Verification items for the finished model (mm, model axes). Coordinates: 2 decimals unless noted, no trailing zeros. Loops run counter-clockwise (first coordinate to the right, second up) from the corner with the lowest first, then second, coordinate; pieces in that order, holes last. Notation, with made-up numbers: (-18.75, -23) - (31.25, -23) arc R20 cw to (31.25, 1) - close; hole circle Ø5 at (41, 14.25). An arc over 180 degrees is marked (long way). One line per item, written item: value. Start each with the question number.
(1) Section check A-A (y = 74.5). Record the boundary of the cut face in (x, z).
(2) Section check C-C (z = 0.45). Record the boundary of the cut face in (x, y).
(3) Thickness scan on probe 1 along X at (y, z) = (70, 0.2); probe 2 along X at (y, z) = (6, 0.6). Record the ranges inside material, lowest first. Write a range as [from, to].
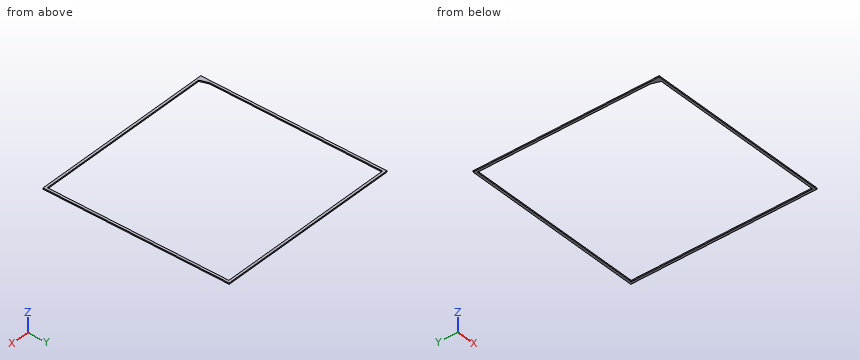
```python
from build123d import *

# Parameters (mm, degrees)
F0_W     = 154
F0_H     = 154
F1_DEPTH = 1


# Not quite as in the source:
# - a feature names something its author has since deleted; it is built from what else it names


with BuildPart() as f1:
    # F0 (on Top) → F1 (new body)
    with BuildSketch(Plane.XY):
        with Locations((75, 75)):
            Rectangle(F0_W, F0_H)
        Polygon((2.3926577996, 0), (0, 0), (0, 7.0679709315), (0, 150), (150, 150), (150, 0), align=None, mode=Mode.SUBTRACT)
        Polygon((0, 7.0679709315), (0, 0), (2.3926577996, 0), align=None)
    extrude(amount=F1_DEPTH)


solid = f1.part
```
Responses:
1. outline: (-2, 0) - (0, 0) - (0, 1) - (-2, 1) - close; (150, 0) - (152, 0) - (152, 1) - (150, 1) - close
2. outline: (-2, -2) - (152, -2) - (152, 152) - (-2, 152) - close; hole (0, 7.07) - (2.39, 0) - (150, 0) - (150, 150) - (0, 150) - close
3. probe 1: x = [-2, 0], [150, 152]
3. probe 2: x = [-2, 0.36], [150, 152]
